Build history of the part. All positions in model axes, mm. A direction names the side the tool comes from. Round coordinates to 2 decimals unless told otherwise and drop trailing zeros. Write each loop counter-clockwise with the first axis right and the second up, starting at its lowest first coordinate (ties: lowest second). Pieces come first, ordered by that corner, then holes. Notation, with made-up numbers: (0, 71) -> (13, 71) arc R14 cw to (13, 86) -> close; hole circle Ø7 at (-16, 84). An arc over 180 degrees is marked (long way). Answer in a Markdown table with one row per item. Add a question column.
from build123d import *

# Parameters (mm, degrees)
SKETCH_1_R               = 1.55
SKETCH_1_R_2             = 1.6
SKETCH_1_W               = 17
SKETCH_1_H               = 3.6
EXTRUDE_1_DEPTH          = 3
HOLE_WIZARD_1_AT_2_COUNT = 2
HOLE_WIZARD_1_AT_2_PITCH = 41.340053217
HOLE_WIZARD_1_AT_3_COUNT = 2
HOLE_WIZARD_1_AT_3_PITCH = 22
HOLE_WIZARD_1_AT_4_COUNT = 2
HOLE_WIZARD_1_AT_4_PITCH = 35
SKETCH_3_W               = 9
SKETCH_3_H               = 5
CUT_EXTRUDE_1_DEPTH      = 10
FILLET_1_R               = 1
SKETCH_4_W               = 16.565491158
SKETCH_4_H               = 15
CUT_EXTRUDE_2_DEPTH      = 10
FILLET_2_R               = 1.5


with BuildPart() as part:
    # 草图1 → 凸台-拉伸1 (new body)
    with BuildSketch(Plane.XY):
        with BuildLine():
            Line((29.5, 20.5), (19.156921938, 20.5))
            Line((19.156921938, 20.5), (15, 13.3))
            Line((15, 13.3), (-15, 13.3))
            Line((-15, 13.3), (-19.156921938, 20.5))
            Line((-19.156921938, 20.5), (-29.5, 20.5))
            Line((-29.5, 20.5), (-23.44914812, -25.679510516))
            ThreePointArc((-23.44914812, -25.679510516), (-17.109416283, -30.887273533), (-11.5, -24.9))
            Line((-11.5, -24.9), (11.5, -24.9))
            ThreePointArc((11.5, -24.9), (17.109416283, -30.887273533), (23.44914812, -25.679510516))
            Line((23.44914812, -25.679510516), (29.5, 20.5))
        make_face()
        with Locations((-24.5, 16.5)):
            Circle(SKETCH_1_R, mode=Mode.SUBTRACT)
        with Locations((-8, -16.5)):
            Circle(SKETCH_1_R_2, mode=Mode.SUBTRACT)
        with Locations(Location((8, -16.5, 0), (0, 0, 180))):
            Circle(SKETCH_1_R_2, mode=Mode.SUBTRACT)
        with Locations(Location((24.5, 16.5, 0), (0, 0, 180))):
            Circle(SKETCH_1_R, mode=Mode.SUBTRACT)
        with Locations((-17.5, -24.9)):
            Circle(SKETCH_1_R, mode=Mode.SUBTRACT)
        with Locations((17.5, -24.9)):
            Circle(SKETCH_1_R, mode=Mode.SUBTRACT)
        with Locations((-17.5, -2.9)):
            Circle(SKETCH_1_R, mode=Mode.SUBTRACT)
        with Locations(Location((17.5, -2.9, 0), (0, 0, 180))):
            Circle(SKETCH_1_R, mode=Mode.SUBTRACT)
        with Locations((0, 8.5)):
            Rectangle(SKETCH_1_W, SKETCH_1_H, mode=Mode.SUBTRACT)
    extrude(amount=EXTRUDE_1_DEPTH)

    # 草图2 → 打孔尺寸(%根据十字)槽沉头木螺钉的类型1 (revolve, cut)
    with BuildSketch(Plane(origin=(-17.5, -24.9, 0), x_dir=(0, 1, 0), z_dir=(1, 0, 0))):
        Polygon((0, 0), (0, 3), (1.55, 3), (1.55, 1.75), (3.3, 0), align=None)
    hole_wizard_1 = revolve(axis=Axis((-17.5, -24.9, -6.35), (0, 0, 1)), mode=Mode.SUBTRACT)

    # 打孔尺寸(%根据十字)槽沉头木螺钉的类型1 at 2: 打孔尺寸(%根据十字)槽沉头木螺钉的类型1 ×2
    with Locations(*[Vector(0.846636549211005, 0.5321715452183458, 0) * (i * HOLE_WIZARD_1_AT_2_PITCH) for i in range(1, HOLE_WIZARD_1_AT_2_COUNT)]):
        add(hole_wizard_1, mode=Mode.SUBTRACT)

    # 打孔尺寸(%根据十字)槽沉头木螺钉的类型1 at 3: 打孔尺寸(%根据十字)槽沉头木螺钉的类型1 ×2
    with Locations(*[(0, i * HOLE_WIZARD_1_AT_3_PITCH, 0) for i in range(1, HOLE_WIZARD_1_AT_3_COUNT)]):
        add(hole_wizard_1, mode=Mode.SUBTRACT)

    # 打孔尺寸(%根据十字)槽沉头木螺钉的类型1 at 4: 打孔尺寸(%根据十字)槽沉头木螺钉的类型1 ×2
    with Locations(*[(i * HOLE_WIZARD_1_AT_4_PITCH, 0, 0) for i in range(1, HOLE_WIZARD_1_AT_4_COUNT)]):
        add(hole_wizard_1, mode=Mode.SUBTRACT)

    # 草图3 → 切除-拉伸1 (cut)
    with BuildSketch(Plane.XY.offset(3)):
        with Locations((29.5, 10)):
            Rectangle(SKETCH_3_W, SKETCH_3_H)
        with Locations((-29.5, 10)):
            Rectangle(SKETCH_3_W, SKETCH_3_H)
    extrude(amount=-CUT_EXTRUDE_1_DEPTH, mode=Mode.SUBTRACT)

    # 圆角1
    fillet_1_edges = [part.edges().sort_by_distance(p)[0] for p in [
        (28.451768555, 12.5, 1.5),
        (27.796623902, 7.5, 1.5),
        (-28.451768555, 12.5, 1.5),
        (-27.796623902, 7.5, 1.5),
        (25, 7.5, 1.5),
        (25, 12.5, 1.5),
        (-25, 12.5, 1.5),
        (-25, 7.5, 1.5),
        (-19.156921938, 20.5, 1.5),
        (-15, 13.3, 1.5),
        (15, 13.3, 1.5),
        (19.156921938, 20.5, 1.5),
        (29.5, 20.5, 1.5),
        (11.5, -24.9, 1.5),
        (-11.5, -24.9, 1.5),
        (-29.5, 20.5, 1.5),
        (8.5, 6.7, 1.5),
        (8.5, 10.3, 1.5),
        (-8.5, 10.3, 1.5),
        (-8.5, 6.7, 1.5),
    ]]
    fillet(fillet_1_edges, radius=FILLET_1_R)

    # 草图4 → 切除-拉伸2 (cut)
    with BuildSketch(Plane(origin=(0, 0, 0), x_dir=(-1, 0, 0), z_dir=(0, 0, -1))):
        with Locations((29.582745579, -23.4)):
            Rectangle(SKETCH_4_W, SKETCH_4_H)
    extrude(amount=-CUT_EXTRUDE_2_DEPTH, mode=Mode.SUBTRACT)

    # 圆角2
    fillet_2_edges = [part.edges().sort_by_distance(p)[0] for p in [
        (-21.3, -29.543274706, 1.5),
        (-24.730546925, -15.9, 1.5),
        (-21.3, -15.9, 1.5),
    ]]
    fillet(fillet_2_edges, radius=FILLET_2_R)


solid = part.part
(1) Which spindle directions (+Z, -Z, +X, -X, +Y, -Y) get a long thin tool onto all of the face, cutting with end or side? Do faces 4 (the face through (-27, 12.5, 2)), 5 (the face through (27, 12.5, 2)), 6 (the face through (8.5, 8, 1)). Say none if no direction does.
(2) Saw through at B-B (y = 16.5). List the corners of the cut face in (x, z).
(3) Probe line 1 along Y through (x, z) = (-8, 1.1); line 2 along X through (y, z) = (-2.9, 2.2); line 3 along X through (y, z) = (-26, 1.65). List the from-to ranges inside material, lowest first.
(4) Drop flat-ended pins along their axis: P1, Ø2.5, axis at x = -8, y = -16.5, coming from the +Z side; P2, Ø0.8, axis at y = 9, z = 1.5, coming from the -X side; P3, Ø5, axis at x = 17.5, y = -2.9, coming from the -Z side; P4, Ø1.5, axis at y = -14.5, z = 1, coming from the +X side. Give the stop position or say it passes through.
(5) Saw through at A-A (x = 5.5). List the corners of the cut face in (y, z).
(6) Saw through at C-C (x = 17.5). List the corners of the cut face in (y, z).
(7) Mould opens along Y. For faces 1 (the face through (-26.294, -3.966, 1.479)), 2 (the face through (-24.702, 18.037, 1.479)), 3 (the face through (-17.053, 16.857, 1.479)) say: pulls with the +Y half, pulls with the -Y half, needs draft (parallel to the pull), parting line crosses it, or undercut.
(8) Saw through at D-D (y = -2.9). List the corners of the cut face in (x, z).
Answer sheet:
| question | item | result |
|---|---|---|
| 1 | face 4 | +Z, -Z, -X |
| 1 | face 5 | +Z, -Z, +X |
| 1 | face 6 | +Z, -Z |
| 2 | outline | (-28.98, 0) -> (-26.05, 0) -> (-26.05, 3) -> (-28.98, 3) -> close; (-22.95, 0) -> (-16.85, 0) -> (-16.85, 3) -> (-22.95, 3) -> close; (16.85, 0) -> (22.95, 0) -> (22.95, 3) -> (16.85, 3) -> close; (26.05, 0) -> (28.98, 0) -> (28.98, 3) -> (26.05, 3) -> close |
| 3 | line 1 | y = -24.9 to -18.1, -14.9 to 6.83, 10.17 to 13.3 |
| 3 | line 2 | x = -26.43 to -19.05, -15.95 to 15.95, 19.05 to 26.43 |
| 3 | line 3 | x = -21.3 to -18.73, -16.27 to -11.6, 11.6 to 16.27, 18.73 to 23.4 |
| 4 | P1 | passes through |
| 4 | P2 | stops at x = -25 |
| 4 | P3 | stops at z = 0.8 |
| 4 | P4 | stops at x = 25.01 |
| 5 | outline | (-24.9, 0) -> (6.7, 0) -> (6.7, 3) -> (-24.9, 3) -> close; (10.3, 0) -> (13.3, 0) -> (13.3, 3) -> (10.3, 3) -> close |
| 6 | outline | (-30.9, 0) -> (-28.2, 0) -> (-26.45, 1.75) -> (-26.45, 3) -> (-30.9, 3) -> close; (-23.35, 1.75) -> (-21.6, 0) -> (-6.2, 0) -> (-4.45, 1.75) -> (-4.45, 3) -> (-23.35, 3) -> close; (-1.35, 1.75) -> (0.4, 0) -> (17.63, 0) -> (17.63, 3) -> (-1.35, 3) -> close |
| 7 | face 1 | pulls with the -Y half |
| 7 | face 2 | undercut |
| 7 | face 3 | pulls with the +Y half |
| 8 | outline | (-26.43, 0) -> (-20.8, 0) -> (-19.05, 1.75) -> (-19.05, 3) -> (-26.43, 3) -> close; (-15.95, 1.75) -> (-14.2, 0) -> (14.2, 0) -> (15.95, 1.75) -> (15.95, 3) -> (-15.95, 3) -> close; (19.05, 1.75) -> (20.8, 0) -> (26.43, 0) -> (26.43, 3) -> (19.05, 3) -> close |
